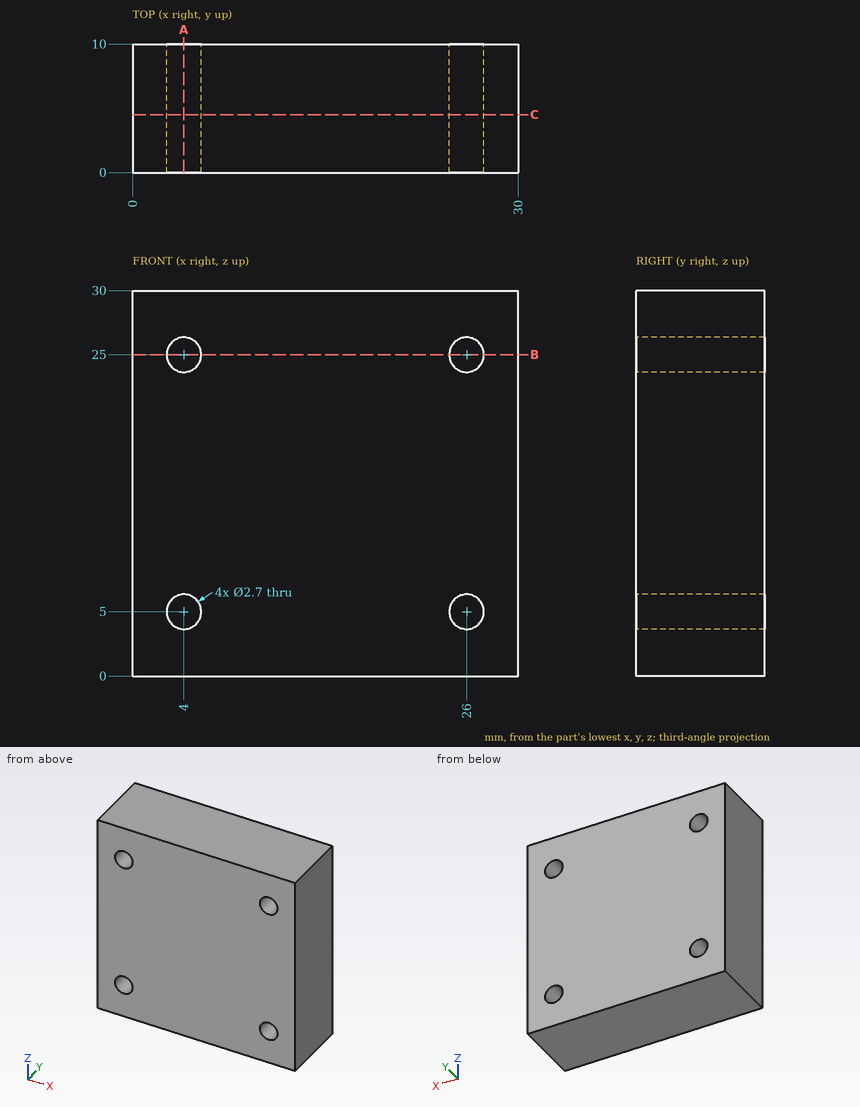
Study the drawing (mm; zero at the part's minimum x, y, z) and answer. Give positions to 0.01 mm unless a question says otherwise; leave off trailing zeros. Order: outer loops, then holes, each group sorted by start corner. A loop starts at its lowest first (then second) coordinate and runs counter-clockwise, first axis right, second up. Notation, with made-up numbers: M -26.5,22 L 26.5,22 A19 cw 26.5,27 Z; hole C 38,31 d7. An arc over 180 degrees is marked long. Put each result on its own line as item: value. Start each with the question number.
Item 1: The part is cut by section C-C, the plane y = 4.5. Determine the outline of the cut face in (x, z).
Item 2: Find the intervals of material crossed by line 1 along X through (y, z) = (7.25, 5); line 2 along Z through (x, y) = (4, 8); line 3 along X through (y, z) = (7.75, 24.25), in increasing order.
Item 3: The part is cut by section A-A, the plane x = 4. Determine the outline of the cut face in (y, z), and give its area (3 significant figures).
Item 4: The part is cut by section B-B, the plane z = 25. Determine the outline of the cut face in (x, y), and give its area (3 significant figures).
Item 5: A flat-ended cylindrical pin translates along its axis: P1, Ø2.5, axis at x = 26, z = 5, coming from the +Y side. Find the tip coordinate at first contact, or state that the pin passes through.
Answer key:
1. outline: M 0,0 L 30,0 L 30,30 L 0,30 Z; hole C 4,5 d2.7; hole C 4,25 d2.7; hole C 26,5 d2.7; hole C 26,25 d2.7
2. line 1: x = 0 to 2.65, 5.35 to 24.65, 27.35 to 30
2. line 2: z = 0 to 3.65, 6.35 to 23.65, 26.35 to 30
2. line 3: x = 0 to 2.88, 5.12 to 24.88, 27.12 to 30
3. outline: M 0,0 L 10,0 L 10,3.65 L 0,3.65 Z; M 0,6.35 L 10,6.35 L 10,23.65 L 0,23.65 Z; M 0,26.35 L 10,26.35 L 10,30 L 0,30 Z
3. area: 246 mm²
4. outline: M 0,0 L 2.65,0 L 2.65,10 L 0,10 Z; M 5.35,0 L 24.65,0 L 24.65,10 L 5.35,10 Z; M 27.35,0 L 30,0 L 30,10 L 27.35,10 Z
4. area: 246 mm²
5. P1: passes through
